from build123d import *

# Parameters (mm, degrees)
SKETCH1_R                  = 30
BOSS_EXTRUDE1_DEPTH        = 4
SKETCH2_R                  = 12
BOSS_EXTRUDE2_DEPTH        = 16
F_4_0_4_DIAMETER_HOLE1_D   = 4
F_10_0_10_DIAMETER_HOLE1_D = 10
SKETCH7_W                  = 2
SKETCH7_H                  = 24


with BuildPart() as part:
    # Sketch1 → Boss-Extrude1 (new body)
    with BuildSketch(Plane.XY):
        with Locations(Location((0, 0, 0), (0, 0, 180))):
            Circle(SKETCH1_R)
    extrude(amount=-BOSS_EXTRUDE1_DEPTH)

    # Sketch2 → Boss-Extrude2 (add)
    with BuildSketch(Plane.XY):
        with Locations(Location((0, 0, 0), (0, 0, 180))):
            Circle(SKETCH2_R)
    extrude(amount=BOSS_EXTRUDE2_DEPTH)

    # Ø4.0 (4) Diameter Hole1 (through all)
    with Locations(Plane.XY):
        with Locations((20.56810334, -11.875), (0, 23.75), (0, -23.75), (20.56810334, 11.875), (-20.56810334, 11.875), (-20.56810334, -11.875)):
            Hole(F_4_0_4_DIAMETER_HOLE1_D / 2)

    # Ø10.0 (10) Diameter Hole1 (through all)
    with Locations(Plane.XY.offset(16)):
        with Locations((0, 0)):
            Hole(F_10_0_10_DIAMETER_HOLE1_D / 2)

    # Sketch7 → Ø4.0 (4) Diameter Hole2 (revolve, cut)
    with BuildSketch(Plane(origin=(0, -4.582575695, 8), x_dir=(0, 0, 1), z_dir=(1, 0, 0))):
        with Locations((1, 12)):
            Rectangle(SKETCH7_W, SKETCH7_H)
    revolve(axis=Axis((0, 1.767424305, 8), (0, -1, 0)), mode=Mode.SUBTRACT)


solid = part.part
Design review of the part built by this model. Coordinates are the model's own, in mm. A direction names the side the tool comes from. Coordinates: 2 decimals unless noted, no trailing zeros. Order: outer loops, then holes, each group sorted by start corner. A loop starts at its lowest first (then second) coordinate and runs counter-clockwise, first axis right, second up. Notation, with made-up numbers: (25, 21.5) - (44, 21.5) arc R29 cw to (44, 54.5) - close; hole circle Ø8 at (-15, -34). An arc over 180 degrees is marked (long way). Put each result on its own line as item: value.
1) The part is to be moulded in two halves that separate along X. For faces 1 (the face through (-5.2, -0.2, 16)), 2 (the face through (-5.537, 10.646, 7.888)), 3 (the face through (0.26, -21.767, -2.028)), say which applies: released by +X, released by -X, zero draft, split by the parting line, or undercut.
Response values:
face 1: zero draft
face 2: split by the parting line
face 3: undercut
2) Insertion check: P1, Ø2.5, axis at x = 0, y = -23.75, coming from the +Z side; P2, Ø5, axis at y = 7, z = 4, coming from the -X side; P3, Ø10, axis at x = -10, y = 12, coming from the +Z side; P4, Ø5, axis at x = 0, z = 8, coming from the -Y side. Each pin has a flat end and moves straight along its axis. Give the tip position at first contact, or say it passes through.
Response values:
P1: passes through
P2: stops at x = -11.12
P3: stops at z = 16
P4: stops at y = -12
3) Wall thickness on L1, parallel to Y at x = 0, z = -2.75; L2, parallel to Z at x = 20.5, y = -18; L3, parallel to X at y = -23.5, z = -0.75: over which ranges is each line inside the solid? List them lowest first. Write a range as from..to.
Response values:
L1: y = -30..-25.75, -21.75..-5, 5..21.75, 25.75..30
L2: z = -4..0
L3: x = -18.65..-1.98, 1.98..18.65
4) Take a section at C-C, the plane z = -2.5. Give the boundary of the cut face in (x, y) (3 decimals).
Response values:
outline: circle Ø60 at (0, 0); hole circle Ø4 at (-20.568, -11.875); hole circle Ø4 at (-20.568, 11.875); hole circle Ø10 at (0, 0); hole circle Ø4 at (0, -23.75); hole circle Ø4 at (0, 23.75); hole circle Ø4 at (20.568, -11.875); hole circle Ø4 at (20.568, 11.875)
5) Tool access review of faces 4 (the face through (-13, 0, 0)), 5 (the face through (18.66, 12.48, -2.03)), 6 (the face through (0, -8, 6)): name each direction out of +Z, -Z, +X, -X, +Y, -Y from which nothing blocks a thin tool from reaching the whole face with its end or side.
Response values:
face 4: +Z
face 5: +Z, -Z
face 6: -Y
6) Take a section at B-B, the plane y = 0. Give the boundary of the cut face in (x, z), and give its area (3 significant figures).
Response values:
outline: (-30, -4) - (-5, -4) - (-5, 16) - (-12, 16) - (-12, 0) - (-30, 0) - close; (5, -4) - (30, -4) - (30, 0) - (12, 0) - (12, 16) - (5, 16) - close
area: 424 mm²
7) Take a section at A-A, the plane x = 0. Give the boundary of the cut face in (y, z), and give its area (3 significant figures).
Response values:
outline: (-30, -4) - (-25.75, -4) - (-25.75, 0) - (-30, 0) - close; (-21.75, -4) - (-5, -4) - (-5, 6) - (-12, 6) - (-12, 0) - (-21.75, 0) - close; (-12, 10) - (-5, 10) - (-5, 16) - (-12, 16) - close; (5, -4) - (21.75, -4) - (21.75, 0) - (12, 0) - (12, 16) - (5, 16) - close; (25.75, -4) - (30, -4) - (30, 0) - (25.75, 0) - close
area: 364 mm²
8) Take a section at D-D, the plane y = -9. Give the boundary of the cut face in (x, z), and give its area (3 significant figures).
Response values:
outline: (-28.62, -4) - (28.62, -4) - (28.62, 0) - (7.94, 0) - (7.94, 16) - (-7.94, 16) - (-7.94, 0) - (-28.62, 0) - close; hole circle Ø4 at (0, 8)
area: 470 mm²
